Source: three-view drawing plus pictorial views. Frame: mm from the lowest corner of the part. Give positions to 0.01 mm unless a question says otherwise; leave off trailing zeros. Write each loop counter-clockwise with the first axis right and the second up, starting at its lowest first coordinate (ties: lowest second). Pieces come first, ordered by that corner, then holes. Notation, with made-up numbers: M -26,-12 L 3,-12 A15 ccw 3,15 Z; hole C 36.25,12.25 d6. An arc over 180 degrees is marked long. One line per question, with ' | ' between items.
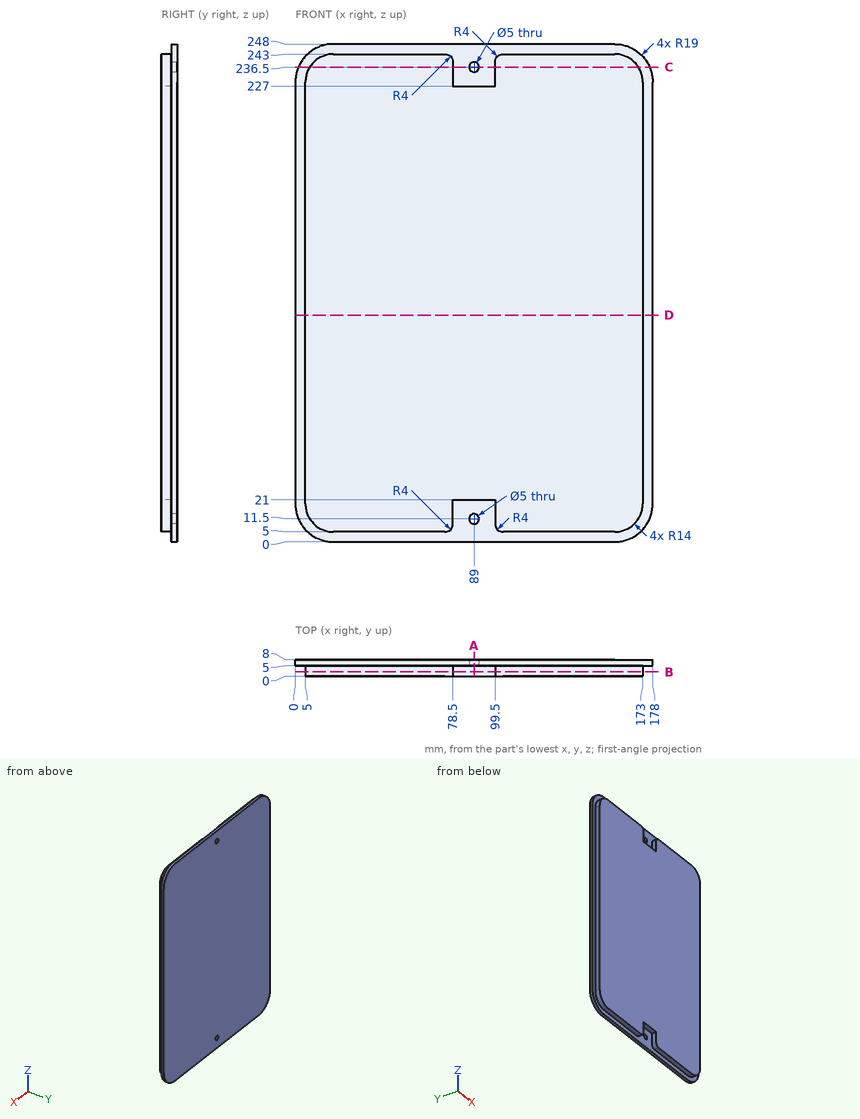
(1) First-contact query: P1, Ø2.5, axis at x = 143, y = 3, coming from the -Z side; P2, Ø4, axis at y = 2, z = 157.5, coming from the -X side; P3, Ø2.5, axis at x = 57, y = 1.5, coming from the +Z side; P4, Ø3, axis at x = 65, y = 5.5, coming from the -Z side. Flat tips, straight axial feed; report the tip coordinate or a pass-through.
Working result:
P1: stops at z = 5 | P2: stops at x = 5 | P3: stops at z = 243 | P4: stops at z = 0
(2) Cut plane C-C, the plane z = 236.5. Return loops of the section in (x, y).
Working result:
outline: M 1.54,5 L 7.18,5 L 7.18,0 L 78.5,0 L 78.5,5 L 86.5,5 L 86.5,8 L 1.54,8 Z; M 91.5,5 L 99.5,5 L 99.5,0 L 170.82,0 L 170.82,5 L 176.46,5 L 176.46,8 L 91.5,8 Z
(3) Material intervals for L1, parallel to Z at x = 89, y = 5.7; L2, parallel to X at y = 3, z = 208; L3, parallel to Z at x = 156.5, y = 2, sorted ascending. Write a range as [from, to].
Working result:
L1: z = [0, 9], [14, 234], [239, 248] | L2: x = [5, 173] | L3: z = [5, 243]
(4) Cut plane B-B, the plane y = 2. Return loops of the section in (x, z), then the cut area to 3 significant figures.
Working result:
outline: M 5,19 A14 ccw 19,5 L 74.5,5 A4 ccw 78.5,9 L 78.5,21 L 99.5,21 L 99.5,9 A4 ccw 103.5,5 L 159,5 A14 ccw 173,19 L 173,229 A14 ccw 159,243 L 103.5,243 A4 ccw 99.5,239 L 99.5,227 L 78.5,227 L 78.5,239 A4 ccw 74.5,243 L 19,243 A14 ccw 5,229 Z | area: 39,100 mm^2
(5) Cut plane A-A, the plane x = 89. Return loops of the section in (y, z).
Working result:
outline: M 0,21 L 5,21 L 5,14 L 8,14 L 8,234 L 5,234 L 5,227 L 0,227 Z; M 5,0 L 8,0 L 8,9 L 5,9 Z; M 5,239 L 8,239 L 8,248 L 5,248 Z
(6) Cut plane D-D, the plane z = 113. Return loops of the section in (x, y), then the cut area to 3 significant figures.
Working result:
outline: M 0,5 L 5,5 L 5,0 L 173,0 L 173,5 L 178,5 L 178,8 L 0,8 Z | area: 1,370 mm^2
